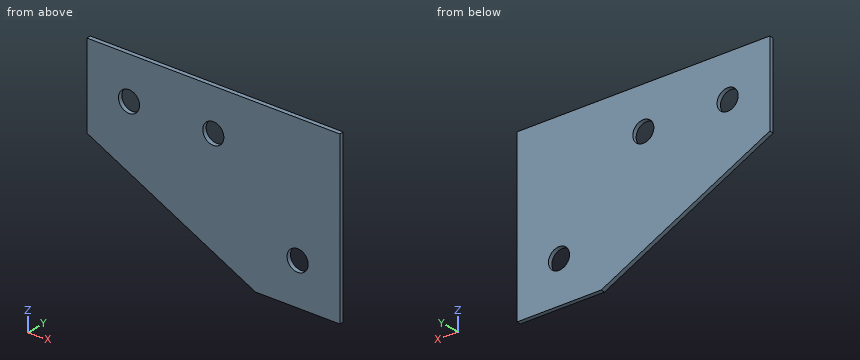
Autodesk Inventor part; units mm, degrees
ref_plane "YZ Plane" through (0, 0, 0) normal (1, 0, 0) x (0, 1, 0)
ref_plane "XZ Plane" through (0, 0, 0) normal (0, 1, 0) x (-1, 0, 0)
ref_plane "XY Plane" through (0, 0, 0) normal (0, 0, 1) x (1, 0, 0)
sketch "Эскиз1" plane through (0, 0, 0) normal (0, 1, 0) x (-1, 0, 0)
  line L0 (0, 0) -> (80, 0)
  line L1 (80, 0) -> (80, -80)
  line L2 (80, -80) -> (0, -80)
  line L3 (0, -80) -> (0, 0)
  line L4 (80, 0) -> (80, -40)
  line L5 (80, -20) -> (60, -20)
  line L6 (40, -80) -> (0, -80)
  line L7 (20, -80) -> (20, -60)
  circle A0 centre (60, -20) radius 5
  circle A1 centre (20, -60) radius 5
  line L8 (80, 0) -> (120, 0)
  line L9 (120, 0) -> (120, -40)
  line L10 (120, -40) -> (80, -40)
  line L11 (80, -40) -> (80, 0)
  line L12 (0, -80) -> (40, -80)
  line L13 (40, -80) -> (120, -40)
  line L14 (80, -20) -> (100, -20)
  circle A2 centre (100, -20) radius 5
  dimension "d0" = 80
  dimension "d1" = 80
  dimension "d2" = 40
  dimension "d3" = 20
  dimension "d4" = 20
  dimension "d5" = 10
  dimension "d6" = 10
  dimension "d7" = 40
  dimension "d8" = 40
  dimension "d9" = 40
  dimension "d10" = 10
extrude "Выдавливание1" add sketch "Эскиз1" along normal blind 2 contours L0 L1 L13 L2 L3 | L8 L9 L10 L1 | L10 L13 L1
properties part number "Угол 80х40"
Geometry: final body of the model. Coordinates: model frame, mm. Coordinates: 2 decimals unless noted, no trailing zeros. Order: outer loops, then holes, each group sorted by start corner. A loop starts at its lowest first (then second) coordinate and runs counter-clockwise, first axis right, second up.
Item 1: Material intervals for line 1 along X through (y, z) = (1.35, -60); line 2 along X through (y, z) = (0.3, -64); line 3 along Z through (x, y) = (-100, 0.9), sorted ascending.
Answer:
line 1: x = -80 to -25, -15 to 0
line 2: x = -72 to -23, -17 to 0
line 3: z = -50 to -25, -15 to 0
Item 2: Section query C-C (z = -20). Output: boundary loops of the cut face in (x, y), then the cut area to 3 significant figures.
Answer:
outline: (-120, 0) - (-105, 0) - (-105, 2) - (-120, 2) - close; (-95, 0) - (-65, 0) - (-65, 2) - (-95, 2) - close; (-55, 0) - (0, 0) - (0, 2) - (-55, 2) - close
area: 200 mm2
Item 3: Section query D-D (y = 1.45). Output: boundary loops of the cut face in (x, z), then the cut area to 3 significant figures.
Answer:
outline: (-120, -40) - (-40, -80) - (0, -80) - (0, 0) - (-120, 0) - close; hole circle Ø10 at (-100, -20); hole circle Ø10 at (-60, -20); hole circle Ø10 at (-20, -60)
area: 7,760 mm2
Item 4: Section query A-A (x = -17). Output: boundary loops of the cut face in (y, z).
Answer:
outline: (0, -80) - (2, -80) - (2, -64) - (0, -64) - close; (0, -56) - (2, -56) - (2, 0) - (0, 0) - close
Item 5: Contact query for a flat-ended pin moving along its axis: P1, Ø10, axis at x = -60.5, z = -20, coming from the -Y side. Output: stop coordinate, or through.
Answer:
P1: stops at y = 0
Item 6: Section query B-B (z = -60). Output: boundary loops of the cut face in (x, y).
Answer:
outline: (-80, 0) - (-25, 0) - (-25, 2) - (-80, 2) - close; (-15, 0) - (0, 0) - (0, 2) - (-15, 2) - close
